Part model, mm, in its own coordinate system. A direction names the side the tool comes from. Give positions to 0.01 mm unless a question says otherwise; leave off trailing zeros. Order: outer loops, then holes, each group sorted by start corner. A loop starts at its lowest first (then second) coordinate and runs counter-clockwise, first axis right, second up.
1. Probe line 1 (Y direction, x = 0, z = 12.5); line 2 (Y direction, x = 0, z = 32); line 3 (Z direction, x = -29.5, y = -22). List the from-to ranges inside material, lowest first.
2. Which spindle directions (+Z, -Z, +X, -X, +Y, -Y) get a long thin tool onto all of the face, cutting with end or side? Do faces 1 (the cylindrical face through (23.9, 37.48, 9.39)), 2 (the cylindrical face through (-30.235, -23.183, 38.278)). Say none if no direction does.
3. Slice it at A-A on y = 0. List the corners of the cut face in (x, z), and give its area (3 significant figures).
4. Slice it at B-B on z = 28. List the corners of the cut face in (x, y).
5. Slice it at D-D on z = 14. List the corners of the cut face in (x, y), and give its area (3 significant figures).
6. Drop flat-ended pins along their axis: pin 1 Ø8 at (y, z) = (12.5, 32) entering from +X; pin 2 Ø8 at (x, z) = (36, 11) entering from +Y; pin 3 Ø1 at (x, z) = (-9, 34.5) entering from +Y. Give the stop position or say it passes through.
7. Mould opens along Y. For faces 3 (the flat face through (-1, 1, 19.05)), 4 (the cylindrical face through (-11.012, -49.592, 18.783)), 5 (the flat face through (0, -45, 0)) say: +Y half, -Y half, draft (parallel to the pull), parting line (faces both ways), or undercut.
from build123d import *

# Parameters (mm, degrees)
F0_R     = 50.8
F1_DEPTH = 50.8
F2_SIZE  = 12.7
F3_DEPTH = 25.4
F4_T     = 6.35


# Not quite as in the source:
# - a shell that OpenCascade refuses in one call is made with other operations: the cavity is built on its own and cut out


with BuildPart() as f1:
    # F0 (on Top) → F1 (new body)
    with BuildSketch(Plane.XY):
        Circle(F0_R)
    extrude(amount=F1_DEPTH)

    # F2
    f2_edges = [f1.edges().sort_by_distance(p)[0] for p in [
        (-50.8, 0, 50.8),
    ]]
    chamfer(f2_edges, length=F2_SIZE)

    # F3 (cut): a face of the model
    f3_faces = [f1.faces().sort_by_distance(p)[0] for p in [
        (0, 0, 50.8),
    ]]
    extrude(f3_faces, amount=-F3_DEPTH, mode=Mode.SUBTRACT)

    # F4: shell of thickness 6.35, made by hand


with BuildPart() as f4_core1:
    # F4_t2: copy of F1
    add(f1.part)

    # the walls: a layer under each face that stays
    f4_faces = [f4_core1.faces().sort_by_distance(p)[0] for p in [
        (-50.8, 0, 19.05),
        (-44.45, 0, 44.45),
        (-38.1, 0, 38.1),
        (0, 0, 25.4),
    ]]
    thicken(f4_faces, amount=-F4_T, mode=Mode.SUBTRACT)

    # F4_s3 → F4_t4 (revolve, cut)
    with BuildSketch(Plane.XZ):
        Polygon((38.0365, 25.4635), (44.45, 25.4), (44.45, 19.05), (38.1, 19.05), align=None)
    revolve(axis=Axis((0, 0, 25.4), (0, 0, 1)), mode=Mode.SUBTRACT)


with BuildPart() as f1_1:
    add(f1.part)

    # what is left inside the walls is the cavity
    f4_cavity = [f4_core1.part.solids().sort_by_distance(p)[0] for p in [
        (0, -14.816667, 18.9865),
    ]]
    add(f4_cavity, mode=Mode.SUBTRACT)


solid = f1_1.part
Data:
1. line 1: y = -50.8 to -44.45, 44.45 to 50.8
1. line 2: y = -50.8 to -38.1, 38.1 to 50.8
1. line 3: z = 19.05 to 25.4
2. face 1: -Z
2. face 2: +Z
3. outline: (-50.8, 0) - (-44.45, 0) - (-44.45, 19.05) - (44.45, 19.05) - (44.45, 0) - (50.8, 0) - (50.8, 38.1) - (38.1, 50.8) - (38.1, 25.4) - (-38.1, 25.4) - (-38.1, 50.8) - (-50.8, 38.1) - close
3. area: 1,370 mm2
4. outline: circle Ø101.6 at (0, 0); hole circle Ø76.2 at (0, 0)
5. outline: circle Ø101.6 at (0, 0); hole circle Ø88.9 at (0, 0)
5. area: 1,900 mm2
6. pin 1: stops at x = 50.08
6. pin 2: stops at y = 39.45
6. pin 3: stops at y = 50.08
7. face 3: undercut
7. face 4: parting line
7. face 5: draft
